Autodesk Inventor part; units mm, degrees
ref_plane "YZ Plane" through (0, 0, 0) normal (1, 0, 0) x (0, 1, 0)
ref_plane "XZ Plane" through (0, 0, 0) normal (0, 1, 0) x (-1, 0, 0)
ref_plane "XY Plane" through (0, 0, 0) normal (0, 0, 1) x (1, 0, 0)
sketch "スケッチ1" plane through (0, 0, 0) normal (0, 0, 1) x (1, 0, 0)
  line L0 (0, 0) -> (98, 0)
  line L1 (98, 0) -> (98, 60)
  line L2 (98, 60) -> (0, 60)
  line L3 (0, 60) -> (0, 0)
  line L4 (98, 0) -> (29, 0)
  line L5 (29, 0) -> (29, 40)
  line L6 (29, 40) -> (98, 40)
  line L7 (98, 40) -> (98, 0)
  line L8 (29, 30) -> (98, 30)
  line L9 (98, 30) -> (98, 10)
  line L10 (98, 10) -> (29, 10)
  line L11 (29, 10) -> (29, 30)
  line L12 (98, 20) -> (0, 20)
  line L13 (29, 20) -> (5.906, 60)
  circle A0 centre (29, 20) radius 8
  circle A1 centre (14, 45.9808) radius 4.05
  line L14 (58, 40) -> (58, 0)
  line L15 (16.8756, 13) -> (-6.2184, 53)
  line L16 (41.1244, 27) -> (18.0303, 67)
  circle A2 centre (14, 45.9808) radius 14
  line L17 (16.8756, 13) -> (25.3526, -1.6825)
  point P0 (58, 30)
  point P1 (33.6188, 40)
  point P2 (22.0718, 60)
  point P3 (0, 45.9808)
  point P4 (1.8756, 38.9808)
  point P5 (24.3812, 0)
  point P6 (58, 0)
  point P7 (58, 10)
  dimension "d0" = 98
  dimension "d1" = 60
  dimension "d2" = 40
  dimension "d3" = 20
  dimension "d4" = 10
  dimension "d5" = 69
  dimension "d6" = 30
  dimension "d7" = 16
  dimension "d8" = 30
  dimension "d9" = 8.1
  dimension "d10" = 40
  dimension "d11" = 28
extrude "押し出し1" add sketch "スケッチ1" along normal blind 5 contours L5 L10 L14 L0 | L0 L17 L15 L12 A0 L5 | L5 A0 L12 L14 L10 | L14 L12 L1 L10 | L14 L8 L1 L12 | L12 A0 L5 L8 L14 | L15 A2 L13 A0 L12 | L8 L16 L6 L14 | A2 L13 A1 | A0 L13 A2 L16 L6 L5 | L8 L5 L6 L16 | L3 L2 L13 A2 | L13 A1 A2 | L13 L2 L16 A2
sketch "スケッチ2" plane through (0, 0, 5) normal (0, 0, 1) x (1, 0, 0)
  line L0 (98, 10) -> (98, 30)
  line L1 (98, 20) -> (47.1161, 20)
  point P0 (0, 0)
  point P1 (88, 20)
  point P2 (58, 20)
  dimension "d14" = 10
  dimension "d15" = 30
hole "穴1" at (88, 20, 5) at (58, 20, 5) direction (0, 0, -1) diameter 3.2 depth 10
fillet "フィレット1" radius 2 6 edges at (58, 40, 2.5) (58, 30, 2.5) (98, 30, 2.5) (98, 10, 2.5) (58, 0, 2.5) (58, 10, 2.5)
fillet "フィレット2" radius 10 4 edges at (24.3812, 0, 2.5) (0, 60, 2.5) (22.0718, 60, 2.5) (33.6188, 40, 2.5)
sketch "スケッチ5" plane through (0, 0, 0) normal (0, 0, -1) x (-1, 0, 0)
  circle A0 centre (-88, 20) radius 1.6
  circle A1 centre (-88, 20) radius 3
  circle A2 centre (-58, 20) radius 1.6
  circle A3 centre (-58, 20) radius 3
  point P0 (0, 0)
  dimension "d38" = 6
  dimension "d39" = 6
extrude "押し出し3" cut sketch "スケッチ5" against normal blind 3 contours A0 | A1 | A2 | A3
sketch "スケッチ6" plane through (0, 0, 0) normal (0, 0, -1) x (-1, 0, 0)
  circle A0 centre (-14, 45.9808) radius 4.05
  circle A1 centre (-14, 45.9808) radius 6.6
  line L0 (-8.4, 49.4736) -> (-8.4, 42.4879)
  arc A2 (-8.4, 47.4736) -> (-8.4, 49.4736) centre (-8.4, 48.4736) ccw
  arc A3 (-8.4, 42.4879) -> (-8.4, 44.4879) centre (-8.4, 43.4879) ccw
  point P0 (0, 0)
  dimension "d42" = 13.2
  dimension "d45" = 5.6
  dimension "d46" = 1
  dimension "d47" = 0
  dimension "d48" = 0
  dimension "d49" = 1
extrude "押し出し4" cut sketch "スケッチ6" against normal blind 2 contours L0 A1 | A2 A1 | A1 A2 L0 | L0 A3 A1 | A1 A3
mirror "ミラー1" about plane through (0, 0, 0) normal (0, 0, 1)
sketch "スケッチ7" plane through (0, 0, 5) normal (0, 0, 1) x (1, 0, 0)
  line L0 (-28.9789, 82.3627) -> (120.5518, 82.3627)
  line L1 (120.5518, 82.3627) -> (120.5518, -18.8106)
  line L2 (120.5518, -18.8106) -> (-28.9789, -18.8106)
  line L3 (-28.9789, -18.8106) -> (-28.9789, 82.3627)
  point P0 (0, 0)
extrude "押し出し5" cut sketch "スケッチ7" against normal blind 5
equation "\"d49\" = d46"
properties part number "RP_Calf-Link-cover-Inside-Left"
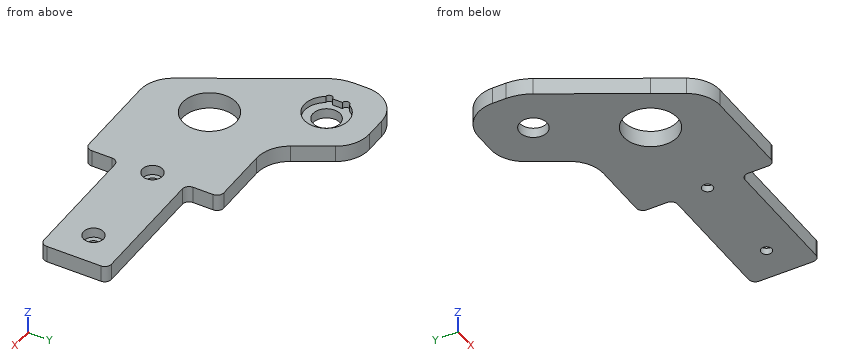
Build history of the part. All positions in model axes, mm. Round coordinates to 2 decimals unless told otherwise and drop trailing zeros. Write each loop counter-clockwise with the first axis right and the second up, starting at its lowest first coordinate (ties: lowest second). Pieces come first, ordered by that corner, then holes. Notation, with made-up numbers: (76.5, -26) - (111.5, -26) arc R9 cw to (111.5, -11) - close; hole circle Ø2 at (40, 47.25). An arc over 180 degrees is marked (long way). Answer as CSV lines item,"result".
Q1. Cut at C-C (z = -4). Write the cut outline in (x, y).
Report:
outline,"(0, 45.98) arc R14 ccw to (1.88, 38.98) - (16.88, 13) - (21.49, 5) arc R10 ccw to (30.15, 0) - (56, 0) arc R2 ccw to (58, 2) - (58, 8) arc R2 cw to (60, 10) - (96, 10) arc R2 ccw to (98, 12) - (98, 28) arc R2 ccw to (96, 30) - (60, 30) arc R2 cw to (58, 32) - (58, 38) arc R2 ccw to (56, 40) - (39.39, 40) arc R10 cw to (30.73, 45) - (24.96, 55) arc R10 ccw to (16.3, 60) - (10, 60) arc R10 ccw to (0, 50) - close; hole circle Ø8.1 at (14, 45.98); hole circle Ø16 at (29, 20); hole circle Ø3.2 at (58, 20); hole circle Ø3.2 at (88, 20)"
Q2. Cut at D-D (y = 43.5). Write the cut outline in (x, z).
Report:
outline,"(0.22, -5) - (10.8, -5) - (10.8, -2) - (7.4, -2) - (7.4, 0) - (0.22, 0) - close; (17.2, -5) - (31.79, -5) - (31.79, 0) - (20.12, 0) - (20.12, -2) - (17.2, -2) - close"
Q3. Cut at B-B (y = 20). Write the cut outline in (x, z).
Report:
outline,"(12.83, -5) - (21, -5) - (21, 0) - (12.83, 0) - close; (37, -5) - (56.4, -5) - (56.4, -3) - (55, -3) - (55, 0) - (37, 0) - close; (59.6, -5) - (86.4, -5) - (86.4, -3) - (85, -3) - (85, 0) - (61, 0) - (61, -3) - (59.6, -3) - close; (89.6, -5) - (98, -5) - (98, 0) - (91, 0) - (91, -3) - (89.6, -3) - close"
Q4. Drop flat-ended pins along their axis: pin 1 (3 mm diameter, centred on y = 32.5, z = -4.5, fed in from -X); pin 2 (1.5 mm diameter, centred on y = 47.5, z = -3.5, fed in from +X); pin 3 (1.5 mm diameter, centred on x = 84.5, z = -3.5, fed in from +Y). Give the stop position or say it passes through.
Report:
pin 1,"stops at x = 4.75"
pin 2,"stops at x = 29.72"
pin 3,"stops at y = 30"
Q5. Cut at A-A (x = 88). Write the cut outline in (y, z), and give its area (3 significant figures).
Report:
outline,"(10, -5) - (18.4, -5) - (18.4, -3) - (17, -3) - (17, 0) - (10, 0) - close; (21.6, -5) - (30, -5) - (30, 0) - (23, 0) - (23, -3) - (21.6, -3) - close"
area,"75.6 mm^2"
Q6. Drill centre lines: probe 1 along X at (y, z) = (20, -3.95); probe 2 along Y at (x, z) = (70, -1.45); probe 3 along X at (y, z) = (20.5, -0.9). Where is each one in solid material? Low to high. Write a range as [from, to].
Report:
probe 1,"x = [12.83, 21], [37, 56.4], [59.6, 86.4], [89.6, 98]"
probe 2,"y = [10, 30]"
probe 3,"x = [12.55, 21.02], [36.98, 55.04], [60.96, 85.04], [90.96, 98]"
